Geometry check sheet. Reference: the model listing, model coordinates, mm. Round coordinates to 2 decimals unless told otherwise and drop trailing zeros. Write each loop counter-clockwise with the first axis right and the second up, starting at its lowest first coordinate (ties: lowest second). Pieces come first, ordered by that corner, then holes. Notation, with made-up numbers: (-6, -3.75) - (6, -3.75) arc R25 ccw to (6, 15.25) - close; hole circle Ø9 at (52.25, -10.75). An arc over 180 degrees is marked (long way). Return JSON: item names as keys, results as strings. Group by question number.
from build123d import *

# Parameters (mm, degrees)
SKETCH1_R           = 4.2
BOSS_EXTRUDE1_DEPTH = 2
CHAMFER1_SIZE       = 0.3


with BuildPart() as part:
    # Sketch1 → Boss-Extrude1 (new body)
    with BuildSketch(Plane(origin=(0, 0, 0), x_dir=(1, 0, 0), z_dir=(0, 1, 0))):
        Polygon((0, 6.350852961), (-5.5, 3.175426481), (-5.5, -3.175426481), (0, -6.350852961), (5.5, -3.175426481), (5.5, 3.175426481), align=None)
        with Locations(Location((0, 0, 0), (0, 0, 270))):
            Circle(SKETCH1_R, mode=Mode.SUBTRACT)
    extrude(amount=BOSS_EXTRUDE1_DEPTH)

    # Chamfer1
    chamfer1_edges = [part.edges().sort_by_distance(p)[0] for p in [
        (0, 0, -4.2),
        (0, 2, -4.2),
    ]]
    chamfer(chamfer1_edges, length=CHAMFER1_SIZE)

    # Sketch3 → Cut-Revolve1 (revolve, cut)
    with BuildSketch(Plane(origin=(0, 0, 0), x_dir=(0, 0, -1), z_dir=(1, 0, 0))):
        Polygon((-6.350852961, 0), (-5.550852961, 0), (-6.350852961, 0.3), align=None)
        Polygon((-6.350852961, 2), (-6.350852961, 1.7), (-5.550852961, 2), align=None)
    revolve(axis=Axis((0, 0, 0), (0, 1, 0)), mode=Mode.SUBTRACT)


solid = part.part
1. Material ranges on line 1 along X through (y, z) = (0.7, 0); line 2 along X through (y, z) = (1.5, 1.75); line 3 along Z through (x, y) = (-0.25, 1.65), recorded low to high.
2. Depth check by flat-ended pin: pin 1 Ø1.5 at (x, z) = (-1, 3) entering from +Y. Enter the tip coordinate at first touch or a pass-through.
3. Section check B-B (y = 1.45). Enter the section's corners in (x, z), and give its area (3 significant figures).
4. Section check A-A (z = 0). Enter the section's corners in (x, y).
5. Mould release check, pull along Z, two halves, no side actions. Record for faces 1 (the face through (-0.031, 0.085, 5.779)), 2 (the face through (1.262, 0.99, 4.006)), 3 (the face through (-2.712, 0.986, -4.785)): pulls with the +Z half, pulls with the -Z half, needs draft (parallel to the pull), parting line crosses it, or undercut.
Result sheet:
{
 "1": {"line 1": "x = -5.5 to -4.2, 4.2 to 5.5", "line 2": "x = -5.5 to -3.82, 3.82 to 5.5", "line 3": "z = -6.21 to -4.19, 4.19 to 6.21"},
 "2": {"pin 1": "passes through"},
 "3": {"outline": "(-5.5, -3.18) - (0, -6.35) - (5.5, -3.18) - (5.5, 3.18) - (0, 6.35) - (-5.5, 3.18) - close; hole circle Ø8.4 at (0, 0)", "area": "49.4 mm²"},
 "4": {"outline": "(-5.5, 0) - (-4.5, 0) - (-4.2, 0.3) - (-4.2, 1.7) - (-4.5, 2) - (-5.5, 2) - close; (4.2, 0.3) - (4.5, 0) - (5.5, 0) - (5.5, 2) - (4.5, 2) - (4.2, 1.7) - close"},
 "5": {"face 1": "pulls with the +Z half", "face 2": "undercut", "face 3": "pulls with the -Z half"}
}
